Geometry check sheet. Reference: the model listing, model coordinates, mm. A direction names the side the tool comes from. Give positions to 0.01 mm unless a question says otherwise; leave off trailing zeros. Loops run counter-clockwise (first coordinate to the right, second up) from the corner with the lowest first, then second, coordinate; pieces in that order, holes last. Notation, with made-up numbers: (9, 10.5) -> (42, 10.5) arc R23 ccw to (42, 43.5) -> close; hole circle Ø1 at (58.25, 60). An arc over 180 degrees is marked (long way). Answer as a JSON object with one key per item and string values.
from build123d import *

# Parameters (mm, degrees)
SKETCH_1_W      = 85
SKETCH_1_H      = 13
SKETCH_1_R      = 2.55
SKETCH_1_W_2    = 7.8
SKETCH_1_H_2    = 4.8
SKETCH_1_W_3    = 7.6
SKETCH_1_H_3    = 3
SKETCH_1_W_4    = 11.2
SKETCH_1_H_4    = 3.7
EXTRUDE_5_DEPTH = 2


with BuildPart() as part:
    # 草图1 → 凸台-拉伸5 (new body)
    with BuildSketch(Plane(origin=(0, 0, 0), x_dir=(1, 0, 0), z_dir=(0, 1, 0))):
        with Locations((32.448630137, -2.468848032)):
            Rectangle(SKETCH_1_W, SKETCH_1_H)
        with Locations(Location((39.591348171, -2.668848032, 0), (0, 0, 270))):
            Circle(SKETCH_1_R, mode=Mode.SUBTRACT)
        with Locations((64.891348171, -2.768848032)):
            Rectangle(SKETCH_1_W_2, SKETCH_1_H_2, mode=Mode.SUBTRACT)
        with Locations((52.191348171, -2.468848032)):
            Rectangle(SKETCH_1_W_3, SKETCH_1_H_3, mode=Mode.SUBTRACT)
        with Locations((24.191348171, -1.018848032)):
            Rectangle(SKETCH_1_W_4, SKETCH_1_H_4, mode=Mode.SUBTRACT)
        with Locations((7.591348171, -1.018848032)):
            Rectangle(SKETCH_1_W_4, SKETCH_1_H_4, mode=Mode.SUBTRACT)
    extrude(amount=EXTRUDE_5_DEPTH)


solid = part.part
1) Section check B-B on x = 53. Record the cut outline in (y, z), plus the area to 3 significant figures.
Geometry check:
{"outline": "(0, -4.03) -> (2, -4.03) -> (2, 0.97) -> (0, 0.97) -> close; (0, 3.97) -> (2, 3.97) -> (2, 8.97) -> (0, 8.97) -> close", "area": "20.0 mm2"}
2) Section check C-C on y = 0.85. Record the cut outline in (x, z), plus the area to 3 significant figures.
Geometry check:
{"outline": "(-10.05, -4.03) -> (74.95, -4.03) -> (74.95, 8.97) -> (-10.05, 8.97) -> close; hole (1.99, -0.83) -> (13.19, -0.83) -> (13.19, 2.87) -> (1.99, 2.87) -> close; hole (18.59, -0.83) -> (29.79, -0.83) -> (29.79, 2.87) -> (18.59, 2.87) -> close; hole circle Ø5.1 at (39.59, 2.67); hole (48.39, 0.97) -> (55.99, 0.97) -> (55.99, 3.97) -> (48.39, 3.97) -> close; hole (60.99, 0.37) -> (68.79, 0.37) -> (68.79, 5.17) -> (60.99, 5.17) -> close", "area": "941 mm2"}
3) Material ranges on line 1 along X through (y, z) = (1.3, -0.25); line 2 along Z through (x, y) = (7, 0.1); line 3 along Z through (x, y) = (52.5, 1.3), recorded low to high. Write a range as from..to.
Geometry check:
{"line 1": "x = -10.05..1.99, 13.19..18.59, 29.79..74.95", "line 2": "z = -4.03..-0.83, 2.87..8.97", "line 3": "z = -4.03..0.97, 3.97..8.97"}
4) Draft check along X on faces 3 (the face through (74.949, 1, 3)), 4 (the face through (32, 2, 2)), 5 (the face through (13.191, 1, 1)). Enter one of: pulls with the +X half, pulls with the -X half, needs draft (parallel to the pull), parting line crosses it, or undercut.
Geometry check:
{"face 3": "pulls with the +X half", "face 4": "needs draft", "face 5": "undercut"}
5) Section check A-A on x = 64. Record the cut outline in (y, z), plus the area to 3 significant figures.
Geometry check:
{"outline": "(0, -4.03) -> (2, -4.03) -> (2, 0.37) -> (0, 0.37) -> close; (0, 5.17) -> (2, 5.17) -> (2, 8.97) -> (0, 8.97) -> close", "area": "16.4 mm2"}
6) Tool access check on faces 1 (the face through (32, 1, 8.969)), 2 (the face through (55.991, 1, 2)). Record the directions out of +Z, -Z, +X, -X, +Y, -Y that give a thin tool (end or side, any length) a straight path to the whole face; none if there is none.
Geometry check:
{"face 1": "+Z, +X, -X, +Y, -Y", "face 2": "+Y, -Y"}
